```python
from build123d import *

# Parameters (mm, degrees)
SKETCH1_W           = 37
SKETCH1_H           = 20
SKETCH1_R           = 1.6
SKETCH1_R_2         = 1.85
BOSS_EXTRUDE1_DEPTH = 5
SKETCH2_W           = 60
SKETCH2_H           = 25
SKETCH2_R           = 1.55
BOSS_EXTRUDE2_DEPTH = 5


with BuildPart() as part:
    # Sketch1 → Boss-Extrude1 (new body)
    with BuildSketch(Plane(origin=(0, 0, 0), x_dir=(1, 0, 0), z_dir=(0, 1, 0))):
        Polygon((-70, 30), (-70, 20), (-104, 20), (-104, -20), (-70, -20), (-70, -30), (70, -30), (70, -20), (104, -20), (104, 20), (70, 20), (70, 30), align=None)
        Rectangle(SKETCH1_W, SKETCH1_H, mode=Mode.SUBTRACT)
        with Locations((-35, -20)):
            Circle(SKETCH1_R, mode=Mode.SUBTRACT)
        with Locations((-35, 20)):
            Circle(SKETCH1_R, mode=Mode.SUBTRACT)
        with Locations((35, -20)):
            Circle(SKETCH1_R, mode=Mode.SUBTRACT)
        with Locations((35, 20)):
            Circle(SKETCH1_R, mode=Mode.SUBTRACT)
        with Locations((-87, 5)):
            Circle(SKETCH1_R_2, mode=Mode.SUBTRACT)
        with Locations((-87, -5)):
            Circle(SKETCH1_R_2, mode=Mode.SUBTRACT)
        with Locations((-92, 0)):
            Circle(SKETCH1_R_2, mode=Mode.SUBTRACT)
        with Locations((-82, 0)):
            Circle(SKETCH1_R_2, mode=Mode.SUBTRACT)
        with Locations((87, 5)):
            Circle(SKETCH1_R_2, mode=Mode.SUBTRACT)
        with Locations((87, -5)):
            Circle(SKETCH1_R_2, mode=Mode.SUBTRACT)
        with Locations((82, 0)):
            Circle(SKETCH1_R_2, mode=Mode.SUBTRACT)
        with Locations((92, 0)):
            Circle(SKETCH1_R_2, mode=Mode.SUBTRACT)
    extrude(amount=BOSS_EXTRUDE1_DEPTH)

    # Sketch2 → Boss-Extrude2 (add)
    with BuildSketch(Plane(origin=(0, 5, 0), x_dir=(1, 0, 0), z_dir=(0, 1, 0))):
        with Locations((0, 42.5)):
            Rectangle(SKETCH2_W, SKETCH2_H)
        with Locations((20, 45)):
            Circle(SKETCH2_R, mode=Mode.SUBTRACT)
        with Locations((-20, 45)):
            Circle(SKETCH2_R, mode=Mode.SUBTRACT)
        with Locations((0, -42.5)):
            Rectangle(SKETCH2_W, SKETCH2_H)
        with Locations((20, -45)):
            Circle(SKETCH2_R, mode=Mode.SUBTRACT)
        with Locations((-20, -45)):
            Circle(SKETCH2_R, mode=Mode.SUBTRACT)
    extrude(amount=-BOSS_EXTRUDE2_DEPTH)


solid = part.part
```
Work out the finished part from the listing and answer in its coordinate system (mm). A direction names the side the tool comes from. Give positions to 0.01 mm unless a question says otherwise; leave off trailing zeros. Loops run counter-clockwise (first coordinate to the right, second up) from the corner with the lowest first, then second, coordinate; pieces in that order, holes last. Notation, with made-up numbers: (36, 15.25) - (94, 15.25) arc R21 ccw to (94, 30.25) - close; hole circle Ø10 at (19.5, 12.25). An arc over 180 degrees is marked (long way). One line per question, with ' | ' between items.
(1) Straight lines are drawn through the part: probe 1 along Z at (x, y) = (-87, 2.5); probe 2 along Z at (x, y) = (-35, 2); probe 3 along X at (y, z) = (3.6, -5). For each, find the intervals that lie inside material, in ascending order.
Recorded:
probe 1: z = -20 to -6.85, -3.15 to 3.15, 6.85 to 20 | probe 2: z = -30 to -21.6, -18.4 to 18.4, 21.6 to 30 | probe 3: x = -104 to -88.85, -85.15 to -18.5, 18.5 to 85.15, 88.85 to 104
(2) Each of these flat-tipped pins is pushed along its axis until it touches: pin 1 Ø1.5 at (y, z) = (3, 25) entering from -X; pin 2 Ø1.5 at (x, y) = (-95, 2) entering from +Z; pin 3 Ø2.5 at (y, z) = (1.5, -27) entering from +X. Where does it stop, or does it pass through?
Recorded:
pin 1: stops at x = -70 | pin 2: stops at z = 20 | pin 3: stops at x = 70
(3) The part is cut by section B-B (y = 1.6). Count the separate pieces of the cut face and the enclosed holes in it, then the cut area to 3 significant figures.
Recorded:
separate pieces: 1 | enclosed holes: 17 | area: 13,200 mm²
(4) The part is cut by section A-A (x = 4). Write down the section's boundary in (y, z).
Recorded:
outline: (0, -55) - (5, -55) - (5, -10) - (0, -10) - close; (0, 10) - (5, 10) - (5, 55) - (0, 55) - close
(5) The part is cut by section C-C (z = 34). Write down the section's boundary in (x, y), then the cut area to 3 significant figures.
Recorded:
outline: (-30, 0) - (30, 0) - (30, 5) - (-30, 5) - close | area: 300 mm²
(6) A tool of negligible diameter and unlimited length cuts with its end or side. For faces 4 (the face through (-87, 2, -20)), 5 (the face through (-87, 2, 20)), 6 (the face through (50, 2, 30)), from which of +Z, -Z, +X, -X, +Y, -Y can it reach the whole face along a straight path? Write none if from no direction.
Recorded:
face 4: -Z, -X, +Y, -Y | face 5: +Z, -X, +Y, -Y | face 6: +Z, +X, +Y, -Y
(7) The part is cut by section D-D (x = 59). Write down the section's boundary in (y, z).
Recorded:
outline: (0, -30) - (5, -30) - (5, 30) - (0, 30) - close
(8) The mould has two halves that part along X. Classify faces 1 (the face through (-1, 0, -13)), 2 (the face through (70, 2, -25)), 3 (the face through (-85.29, 2.46, 5.71)): +X half, -X half, draft (parallel to the pull), parting line (faces both ways), or undercut.
Recorded:
face 1: draft | face 2: +X half | face 3: undercut
